Model file for the job. Use its own axes, mm. Give positions to 0.01 mm unless a question says otherwise; leave off trailing zeros. Loops run counter-clockwise (first coordinate to the right, second up) from the corner with the lowest first, then second, coordinate; pieces in that order, holes last. Notation, with made-up numbers: M 86.5,-37.5 L 101.5,-37.5 A28 cw 101.5,1.5 Z; hole C 33,0 d2. An arc over 180 degrees is marked long. Answer in a Markdown table with one row per item.
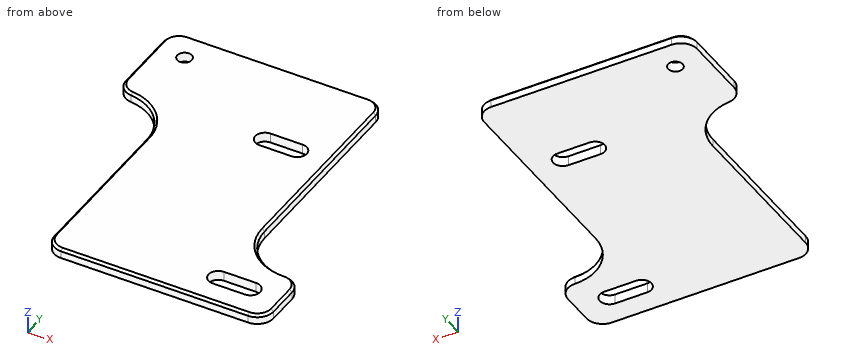
Autodesk Inventor part; units mm, degrees
ref_plane "YZ Plane" through (0, 0, 0) normal (1, 0, 0) x (0, 1, 0)
ref_plane "XZ Plane" through (0, 0, 0) normal (0, 1, 0) x (-1, 0, 0)
ref_plane "XY Plane" through (0, 0, 0) normal (0, 0, 1) x (1, 0, 0)
sketch "Sketch1" plane through (0, 0, 0) normal (0, 0, 1) x (1, 0, 0)
  line L0 (0, 0) -> (-86, 0)
  line L1 (-86, 0) -> (-86, 100)
  line L2 (-86, 100) -> (-20, 100)
  line L3 (-20, 100) -> (-20, 20)
  line L4 (-20, 20) -> (0, 20)
  line L5 (0, 20) -> (0, 0)
  dimension "d0" = 20
  dimension "d1" = 20
  dimension "d2" = 100
  dimension "d3" = 86
extrude "Extrusion1" add sketch "Sketch1" along normal blind 3
sketch "Sketch2" plane through (0, 0, 3) normal (0, 0, 1) x (1, 0, 0)
  line L0 (-86, 0) -> (-68, 0)
  line L1 (-68, 0) -> (-68, 70)
  line L2 (-68, 70) -> (-86, 70)
  line L3 (-86, 70) -> (-86, 0)
  line L4 (-20, 100) -> (-86, 100)
  point P0 (0, 0)
  dimension "d6" = 18
  dimension "d7" = 30
extrude "Extrusion2" cut sketch "Sketch2" against normal blind 3
sketch "Sketch3" plane through (0, 0, 3) normal (0, 0, 1) x (1, 0, 0)
  line L0 (-20, 10) -> (-10, 10) construction
  line L1 (-20, 7) -> (-10, 7)
  line L2 (-10, 13) -> (-20, 13)
  arc A0 (-20, 13) -> (-20, 7) centre (-20, 10) ccw
  arc A1 (-10, 7) -> (-10, 13) centre (-10, 10) ccw
  line L3 (0, 0) -> (0, 20)
  line L4 (0, 20) -> (-20, 20)
  line L5 (-40, 70) -> (-30, 70) construction
  line L6 (-40, 67) -> (-30, 67)
  line L7 (-30, 73) -> (-40, 73)
  arc A2 (-40, 73) -> (-40, 67) centre (-40, 70) ccw
  arc A3 (-30, 67) -> (-30, 73) centre (-30, 70) ccw
  point P0 (-15, 10)
  point P1 (-35, 70)
  dimension "d10" = 15
  dimension "d11" = 10
  dimension "d12" = 3
  dimension "d13" = 10
  dimension "d14" = 20
  dimension "d15" = 3
  dimension "d16" = 10
  dimension "d17" = 60
extrude "Extrusion3" cut sketch "Sketch3" against normal blind 3
fillet "Fillet1" radius 5 6 edges at (0, 0, 1.5) (-68, 0, 1.5) (0, 20, 1.5) (-20, 100, 1.5) (-86, 70, 1.5) (-86, 100, 1.5)
fillet "Fillet1" radius 15 2 edges at (-20, 20, 1.5) (-68, 70, 1.5)
sketch "Sketch4" plane through (0, 0, 3) normal (0, 0, 1) x (1, 0, 0)
  circle A0 centre (-77, 91) radius 2.25
  line L0 (-25, 100) -> (-81, 100)
  line L1 (-86, 95) -> (-86, 75)
  point P0 (0, 0)
  dimension "d22" = 4.5
  dimension "d23" = 9
  dimension "d24" = 9
extrude "Extrusion4" cut sketch "Sketch4" against normal blind 3
chamfer "Chamfer1" distance 0.75 angle 45 14 edges at (-71.8757, 65.1626, 3) (-68, 30.0501, 3) (-66.5355, 1.4645, 3) (-34, 0, 3) (-1.4645, 1.4645, 3) (0, 10, 3) (-1.4645, 18.5355, 3) (-5.0005, 20, 3) (-20, 64.9995, 3) (-21.4645, 98.5355, 3) (-53, 100, 3) (-84.5355, 98.5355, 3) (-86, 85, 3) (-84.7081, 71.6459, 3)
equation "\"d15\" = d12"
equation "\"d16\" = d11"
properties part number "Front"
(1) Wall check: L1, parallel to Y at x = -33, z = 1.65; L2, parallel to X at y = 38, z = 0.7; L3, parallel to X at y = 78, z = 0.2. Give the ranges that are in metal, low to high.
Established:
| item | result |
|---|---|
| L1 | y = 0 to 67, 73 to 100 |
| L2 | x = -68 to -20 |
| L3 | x = -86 to -20 |
(2) Flat gauge pins, fed straight in: P1, Ø1.5, axis at x = -18, z = 1.5, coming from the +Y side; P2, Ø1.5, axis at x = -13.5, z = 1, coming from the +Y side; P3, Ø1, axis at x = -52, y = 49.5, coming from the -Z side; P4, Ø2, axis at x = -70.5, y = 51, coming from the +Z side. Where does each tip first touch, or does it go through?
Established:
| item | result |
|---|---|
| P1 | stops at y = 29 |
| P2 | stops at y = 23.19 |
| P3 | stops at z = 0 |
| P4 | passes through |
(3) Saw through at A-A, the plane x = -34. Give the cut face in (y, z), and give its area (3 significant figures).
Established:
| item | result |
|---|---|
| outline | M 0,0 L 67,0 L 67,3 L 0.75,3 L 0,2.25 Z; M 73,0 L 100,0 L 100,2.25 L 99.25,3 L 73,3 Z |
| area | 281 mm2 |
(4) Saw through at B-B, the plane y = 91. Give the cut face in (x, z), and give its area (3 significant figures).
Established:
| item | result |
|---|---|
| outline | M -86,0 L -79.25,0 L -79.25,3 L -85.25,3 L -86,2.25 Z; M -74.75,0 L -20,0 L -20,2.25 L -20.75,3 L -74.75,3 Z |
| area | 184 mm2 |
(5) Saw through at C-C, the plane z = 1.75. Count the separate pieces of the cut face and the enclosed holes in it, and give its area (3 significant figures).
Established:
| item | result |
|---|---|
| separate pieces | 1 |
| enclosed holes | 3 |
| area | 5,610 mm2 |
